```python
from build123d import *

# Parameters (mm, degrees)
CUT_EXTRUDE1_DEPTH = 1.2
SKETCH6_W          = 17.5
SKETCH6_H          = 1.65
SKETCH7_W          = 26
SKETCH7_H          = 26
CUT_EXTRUDE2_DEPTH = 6.566666667


with BuildPart() as part:
    # Sketch1 → Revolve1 (revolve)
    with BuildSketch(Plane.XY):
        with BuildLine():
            Line((0, 3.675), (3.675, 3.675))
            Line((3.675, 3.675), (5.25, 5.25))
            Line((5.25, 5.25), (12.7, 5.25))
            Line((12.7, 5.25), (13.8, 4.955255888))
            Line((13.8, 4.955255888), (13.8, 4.848076211))
            Line((13.8, 4.848076211), (14.058578644, 4.848076211))
            Line((14.058578644, 4.848076211), (14.2, 4.706654855))
            Line((14.2, 4.706654855), (14.2, 3.5))
            Line((14.2, 3.5), (14.73, 3.5))
            ThreePointArc((14.73, 3.5), (14.991629509, 3.608370491), (15.1, 3.87))
            Line((15.1, 3.87), (15.1, 6.9))
            Line((15.1, 6.9), (15.497402943, 6.9))
            ThreePointArc((15.497402943, 6.9), (15.625960465, 6.853208889), (15.694364494, 6.734729636))
            Line((15.694364494, 6.734729636), (16.3, 3.3))
            Line((16.3, 3.3), (16.3, 0))
            Line((16.3, 0), (-3.675, 0))
            ThreePointArc((-3.675, 0), (-2.598617421, 2.598617421), (0, 3.675))
        make_face()
    revolve(axis=Axis((16.3, 0, 0), (-1, 0, 0)))

    # Sketch2 → Revolve2 (revolve)
    with BuildSketch(Plane(origin=(0, 0, 0), x_dir=(0, 0, -1), z_dir=(1, 0, 0))):
        Polygon((-12.4, 0), (-12.4, 6.3), (-12, 6.3), (-11.9, 6.2), (-11.8, 6.3), (-11.0875, 6.3), (-11.0875, 6.5), (-10.48705572, 7.54), (-6.50669428, 7.54), (-5.90625, 6.5), (-5.90625, 3.9375), (-3.5, 3.9375), (-3.2375, 3.675), (0, 3.675), (0, 0), align=None)
    revolve(axis=Axis((0, 0, 0), (0, 0, 1)))

    # Sketch3 → Revolve3 (revolve)
    with BuildSketch(Plane(origin=(0, 0, 0), x_dir=(0, 0, -1), z_dir=(1, 0, 0))):
        Polygon((-17.5, 0), (-17.5, 4.283), (-16.919, 4.864), (-12.4, 4.864), (-12.4, 0), align=None)
    revolve(axis=Axis((0, 0, 12.4), (0, 0, 1)))

    # Sketch4 → Cut-Extrude1 (cut)
    with BuildSketch(Plane(origin=(16.3, 0, 0), x_dir=(0, 0, -1), z_dir=(1, 0, 0))):
        Polygon((-11.8, -6.812733176), (0, -13.625466353), (11.8, -6.812733176), (11.8, 6.812733176), (0, 13.625466353), (-11.8, 6.812733176), align=None)
        with BuildLine():
            Line((-1, -4.9), (1, -4.9))
            ThreePointArc((1, -4.9), (5.9, 0), (1, 4.9))
            Line((1, 4.9), (-1, 4.9))
            ThreePointArc((-1, 4.9), (-5.9, 0), (-1, -4.9))
        make_face(mode=Mode.SUBTRACT)
    extrude(amount=-CUT_EXTRUDE1_DEPTH, mode=Mode.SUBTRACT)

    # Sketch6 → Cut-Revolve1 (revolve, cut)
    with BuildSketch(Plane(origin=(0, 0, 0), x_dir=(0, 0, -1), z_dir=(1, 0, 0))):
        with Locations((-8.75, 0.825)):
            Rectangle(SKETCH6_W, SKETCH6_H)
    revolve(axis=Axis((0, 0, 0), (0, 0, 1)), mode=Mode.SUBTRACT)

    # Sketch5 → Cut-Revolve2 (revolve, cut)
    with BuildSketch(Plane(origin=(0, 0, 0), x_dir=(1, 0, 0), z_dir=(0, 1, 0))):
        with BuildLine():
            Line((0, 1.65), (4.4, 1.65))
            Line((4.4, 1.65), (4.4, 3))
            Line((4.4, 3), (16, 3))
            ThreePointArc((16, 3), (16.212132034, 3.087867966), (16.3, 3.3))
            Line((16.3, 3.3), (16.3, 0))
            Line((16.3, 0), (-1.65, 0))
            ThreePointArc((-1.65, 0), (-1.166726189, 1.166726189), (0, 1.65))
        make_face()
    revolve(axis=Axis((16.3, 0, 0), (-1, 0, 0)), mode=Mode.SUBTRACT)

    # Sketch7 → Cut-Extrude2 (cut)
    with BuildSketch(Plane.XY.offset(12.4)):
        Rectangle(SKETCH7_W, SKETCH7_H)
        Polygon((-7.505553499, 0), (-3.75277675, -6.5), (3.75277675, -6.5), (7.505553499, 0), (3.75277675, 6.5), (-3.75277675, 6.5), align=None, mode=Mode.SUBTRACT)
    extrude(amount=-CUT_EXTRUDE2_DEPTH, mode=Mode.SUBTRACT)


solid = part.part
```
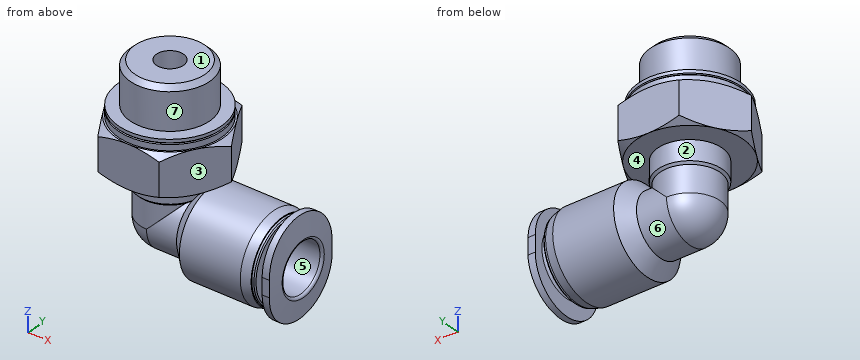
The model under review builds one solid part; all positions refer to its coordinate system, in mm. Face numbers are marked on the shaded views. A direction names the side the tool comes from. Give positions to 0.01 mm unless a question says otherwise; leave off trailing zeros. Write each loop counter-clockwise with the first axis right and the second up, starting at its lowest first coordinate (ties: lowest second). Pieces come first, ordered by that corner, then holes.
(1) To check wall thickness, follow L1, parallel to Y at x = 10, z = 0; L2, parallel to Y at x = 0, z = 12.75. State the ranges of each line that lie inside material, in increasing order.
(2) The part is to be moulded in two halves that separate along Z. For the marked faces 1, 2, 3 and 4, say which applies: released by +Z, released by -Z, zero draft, split by the parting line, or undercut.
(3) Consider section B-B, the plane x = 9. Give the boundary of the cut face in (y, z).
(4) For P1, Ø4, axis at y = 0, z = 0, coming from the -X side (3 decimals); P2, Ø0.5, axis at x = 15.5, z = 0.5, coming from the +Y side; P3, Ø5, axis at x = -3, z = -1, coming from the -Y side, all flat-tipped, find the tip position at first contact; note any pin that passes through.
(5) Consider section A-A, the plane z = 7. Give the boundary of the cut face in (x, y), and give its area (3 significant figures).
(6) Consider section C-C, the plane z = 13.5. Give the boundary of the cut face in (x, y), and give its area (3 significant figures).
(7) Tool access review of the marked faces 5, 6 and 7: name each direction out of +Z, -Z, +X, -X, +Y, -Y from which nothing blocks a thin tool from reaching the whole face with its end or side.
Returned:
1. L1: y = -5.25 to -3, 3 to 5.25
1. L2: y = -4.86 to -1.65, 1.65 to 4.86
2. face 1: released by +Z
2. face 2: undercut
2. face 3: zero draft
2. face 4: undercut
3. outline: circle Ø10.5 at (0, 0); hole circle Ø6 at (0, 0)
4. P1: stops at x = -3.675
4. P2: stops at y = 4.9
4. P3: stops at y = -3.61
5. outline: (-7.51, 0) - (-3.75, -6.5) - (3.75, -6.5) - (7.51, 0) - (3.75, 6.5) - (-3.75, 6.5) - close; hole circle Ø3.3 at (0, 0)
5. area: 138 mm2
6. outline: circle Ø9.73 at (0, 0); hole circle Ø3.3 at (0, 0)
6. area: 65.8 mm2
7. face 5: +X
7. face 6: none
7. face 7: +Z
